Geometry: final body of the model. Coordinates: model frame, mm. Face numbers are marked on the shaded views. A direction names the side the tool comes from. Coordinates: 2 decimals unless noted, no trailing zeros. Loops run counter-clockwise (first coordinate to the right, second up) from the corner with the lowest first, then second, coordinate; pieces in that order, holes last. Notation, with made-up numbers: (39, 48) - (71, 48) arc R10 ccw to (71, 55) - close; hole circle Ø5 at (31.25, 2). An arc over 180 degrees is marked (long way). Return JSON: item names as keys, results as strings.
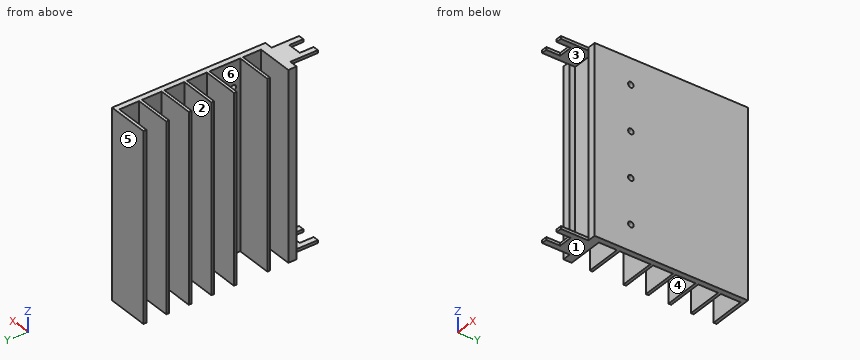
from build123d import *

# Parameters (mm, degrees)
F1_DEPTH = 67.12
F2_DEPTH = 1
F3_START = 66.12
F3_DEPTH = 1
F5_D     = 2


with BuildPart() as f1:
    # F0 (on Top) → F1 (new body)
    with BuildSketch(Plane.XY):
        Polygon((0, 0), (0, 55), (-15, 55), (-15, 54.9), (-15, 53.9), (-2, 53.9), (-2, 46.8), (-15, 46.8), (-15, 45.8), (-2, 45.8), (-2, 38.7), (-15, 38.7), (-15, 37.7), (-2, 37.7), (-2, 30.6), (-15, 30.6), (-15, 29.6), (-2, 29.6), (-2, 22.5), (-15, 22.5), (-15, 21.5), (-2, 21.5), (-2, 10.5), (-15, 10.5), (-15, 9.5), (-2, 9.5), (-2, 3), (-15, 3), (-15, 0), (-12, 0), (-12, 2), (-3, 2), (-3, 0), align=None)
    extrude(amount=F1_DEPTH)

    # F0 (on Top) → F2 (join)
    with BuildSketch(Plane.XY):
        Polygon((-3, -9.87), (-3, 0), (-3, 2), (-12, 2), (-12, 0), (-12, -9.87), (-10, -9.87), (-10, -4.87), (-5, -4.87), (-5, -9.87), align=None)
    extrude(amount=F2_DEPTH)

    # F0 (on Top) → F3 (join)
    with BuildSketch(Plane.XY.offset(F3_START)):
        Polygon((-3, -9.87), (-3, 0), (-3, 2), (-12, 2), (-12, 0), (-12, -9.87), (-10, -9.87), (-10, -4.87), (-5, -4.87), (-5, -9.87), align=None)
    extrude(amount=F3_DEPTH)

    # F5 (through all)
    with Locations(Plane.YZ):
        with Locations((13, 57.87), (13, 41.6633333333), (13, 25.4566666667), (13, 9.25)):
            Hole(F5_D / 2)


solid = f1.part
Item 1: First-contact query: pin 1 Ø0.8 at (y, z) = (-8, 0.5) entering from +X; pin 2 Ø2 at (y, z) = (33, 17) entering from -X; pin 3 Ø4 at (x, z) = (-7.5, 18) entering from -Y. Flat tips, straight axial feed; report the tip coordinate or a pass-through.
Worked out:
{"pin 1": "x = -3", "pin 2": "x = -2", "pin 3": "y = 2"}
Item 2: Reachability of the marked faces 1 and 2 from +Z, -Z, +X, -X, +Y, -Y: full face, straight path, thin tool, end or side. Return the list, or none.
Worked out:
{"face 1": "-Z, +X, -X, +Y, -Y", "face 2": "+Z, -Z, -X"}
Item 3: Ray query, probe 1 along Z at (x, y) = (-0.5, 13); probe 2 along Z at (x, y) = (-11, -2); probe 3 along X at (y, z) = (14.5, 32.5). Return the intervals inside material, ascending. Write a range as from..to.
Worked out:
{"probe 1": "0..8.25, 10.25..24.46, 26.46..40.66, 42.66..56.87, 58.87..67.12", "probe 2": "0..1, 66.12..67.12", "probe 3": "-2..0"}
Item 4: Mould query, pull axis Y, two halves, no side actions, for the marked faces 3, 4, 5 and 6. Classes: +Y half, -Y half, draft (parallel to the pull), parting line (faces both ways), or undercut.
Worked out:
{"face 3": "draft", "face 4": "undercut", "face 5": "+Y half", "face 6": "undercut"}
Item 5: Section query D-D, the plane y = 44.5. Return loops of the section in (x, z).
Worked out:
{"outline": "(-2, 0) - (0, 0) - (0, 67.12) - (-2, 67.12) - close"}
Item 6: Section query B-B, the plane x = -8.25. Count the separate pieces of the cut face and the enclosed holes in it, and give its area (3 significant figures).
Worked out:
{"separate pieces": "7", "enclosed holes": "0", "area": "490 mm^2"}
Item 7: Section query A-A, the plane y = 13. Return loops of the section in (x, z).
Worked out:
{"outline": "(-2, 0) - (0, 0) - (0, 8.25) - (-2, 8.25) - close; (-2, 10.25) - (0, 10.25) - (0, 24.46) - (-2, 24.46) - close; (-2, 26.46) - (0, 26.46) - (0, 40.66) - (-2, 40.66) - close; (-2, 42.66) - (0, 42.66) - (0, 56.87) - (-2, 56.87) - close; (-2, 58.87) - (0, 58.87) - (0, 67.12) - (-2, 67.12) - close"}
